from build123d import *

# Parameters (mm, degrees)
SKETCH1_W                                     = 40
SKETCH1_H                                     = 30
BOSS_EXTRUDE1_DEPTH                           = 10
SKETCH2_W                                     = 4.5
SKETCH2_H                                     = 8
CUT_EXTRUDE1_DEPTH                            = 1
CUT_EXTRUDE2_DEPTH                            = 11
SKETCH4_W                                     = 40
SKETCH4_H                                     = 15.897693
BOSS_EXTRUDE3_DEPTH                           = 15
FIX_DISTANCES_CONVEX_LENS_SEAT_DEPTH          = 3
CHOOSE_SCREW_SIZE_USE_TIGHT_TOLERANCE_C_DEPTH = 16.897693


with BuildPart() as part:
    # Sketch1 → Boss-Extrude1 (new body)
    with BuildSketch(Plane(origin=(0, 0, 0), x_dir=(0, 0, -1), z_dir=(1, 0, 0))):
        with Locations((3.569892473, -6.978494624)):
            Rectangle(SKETCH1_W, SKETCH1_H)
    extrude(amount=BOSS_EXTRUDE1_DEPTH)

    # Sketch2 → Cut-Extrude1 (cut)
    with BuildSketch(Plane.ZY):
        with BuildLine():
            Line((-5.319892473, 2.419198376), (-1.819892473, 2.419198376))
            ThreePointArc((-1.819892473, 2.419198376), (-1.466339083, 2.272751767), (-1.319892473, 1.919198376))
            Line((-1.319892473, 1.919198376), (-5.819892473, 1.919198376))
            ThreePointArc((-5.819892473, 1.919198376), (-5.673445864, 2.272751767), (-5.319892473, 2.419198376))
        make_face()
        with BuildLine():
            Line((-5.319892473, -6.580801624), (-1.819892473, -6.580801624))
            ThreePointArc((-1.819892473, -6.580801624), (-1.466339083, -6.434355014), (-1.319892473, -6.080801624))
            Line((-1.319892473, -6.080801624), (-5.819892473, -6.080801624))
            ThreePointArc((-5.819892473, -6.080801624), (-5.673445864, -6.434355014), (-5.319892473, -6.580801624))
        make_face()
        with Locations((-3.569892473, -2.080801624)):
            Rectangle(SKETCH2_W, SKETCH2_H)
        with BuildLine():
            ThreePointArc((-2.569892473, 2.419198376), (-3.569892473, 3.419198376), (-4.569892473, 2.419198376))
            Line((-4.569892473, 2.419198376), (-2.569892473, 2.419198376))
        make_face()
        with BuildLine():
            Line((-2.569892473, -6.580801624), (-4.569892473, -6.580801624))
            ThreePointArc((-4.569892473, -6.580801624), (-3.569892473, -7.580801624), (-2.569892473, -6.580801624))
        make_face()
    extrude(amount=-CUT_EXTRUDE1_DEPTH, mode=Mode.SUBTRACT)

    # Sketch3 → Cut-Extrude2 (cut, through all)
    with BuildSketch(Plane.ZY):
        with BuildLine():
            Line((-18.069892473, 1.919198376), (10.930107527, 1.919198376))
            ThreePointArc((10.930107527, 1.919198376), (12.69787448, 1.186965329), (13.430107527, -0.580801624))
            Line((13.430107527, -0.580801624), (13.430107527, -3.580801624))
            ThreePointArc((13.430107527, -3.580801624), (12.69787448, -5.348568577), (10.930107527, -6.080801624))
            Line((10.930107527, -6.080801624), (-18.069892473, -6.080801624))
            ThreePointArc((-18.069892473, -6.080801624), (-19.837659426, -5.348568577), (-20.569892473, -3.580801624))
            Line((-20.569892473, -3.580801624), (-20.569892473, -0.580801624))
            ThreePointArc((-20.569892473, -0.580801624), (-19.837659426, 1.186965329), (-18.069892473, 1.919198376))
        make_face()
    extrude(amount=-CUT_EXTRUDE2_DEPTH, mode=Mode.SUBTRACT)

    # Sketch4 → Boss-Extrude3 (add)
    with BuildSketch(Plane(origin=(10, 0, 0), x_dir=(0, 0, -1), z_dir=(1, 0, 0))):
        with Locations((3.569892473, -14.029648124)):
            Rectangle(SKETCH4_W, SKETCH4_H)
    extrude(amount=BOSS_EXTRUDE3_DEPTH)

    # Sketch6 → [fix distances] convex_lens_seat (cut)
    with BuildSketch(Plane(origin=(0, -6.080801624, 0), x_dir=(1, 0, 0), z_dir=(0, 1, 0))):
        Polygon((17, 2.569892473), (17, -1.680107527), (25, -1.680107527), (25, 8.819892473), (17, 8.819892473), (17, 4.569892473), align=None)
        with BuildLine():
            ThreePointArc((17, 4.569892473), (16, 3.569892473), (17, 2.569892473))
            Line((17, 2.569892473), (17, 4.569892473))
        make_face()
    extrude(amount=-FIX_DISTANCES_CONVEX_LENS_SEAT_DEPTH, mode=Mode.SUBTRACT)

    # Sketch7 → [choose screw size, use tight tolerance clearance diameter ] slots (cut, through all)
    with BuildSketch(Plane(origin=(0, -6.080801624, 0), x_dir=(1, 0, 0), z_dir=(0, 1, 0))):
        with BuildLine():
            Line((15.746714751, 12.781776292), (15.746714751, 19.608008654))
            ThreePointArc((15.746714751, 19.608008654), (17.5, 21.361293903), (19.253285249, 19.608008654))
            Line((19.253285249, 19.608008654), (19.253285249, 12.781776292))
            ThreePointArc((19.253285249, 12.781776292), (17.5, 11.028491043), (15.746714751, 12.781776292))
        make_face()
        with BuildLine():
            Line((15.746714751, -5.641991346), (15.746714751, -12.468223708))
            ThreePointArc((15.746714751, -12.468223708), (17.5, -14.221508957), (19.253285249, -12.468223708))
            Line((19.253285249, -12.468223708), (19.253285249, -5.641991346))
            ThreePointArc((19.253285249, -5.641991346), (17.5, -3.888706097), (15.746714751, -5.641991346))
        make_face()
    extrude(amount=-CHOOSE_SCREW_SIZE_USE_TIGHT_TOLERANCE_C_DEPTH, mode=Mode.SUBTRACT)


solid = part.part
Input: part model. Units: mm. Frame: model coordinates. A direction names the side the tool comes from. Give positions to 0.01 mm unless a question says otherwise; leave off trailing zeros. Write each loop counter-clockwise with the first axis right and the second up, starting at its lowest first coordinate (ties: lowest second). Pieces come first, ordered by that corner, then holes. Notation, with made-up numbers: (39, -13.5) -> (98, -13.5) arc R14 cw to (98, 3.5) -> close; hole circle Ø6 at (14, 4.25). An arc over 180 degrees is marked (long way). Use one line per item in the form item = value. Start each with the question number.
1) Section query D-D on z = -9.5. Return the cut outline in (x, y), then the cut area to 3 significant figures.
2) Section query C-C on y = -18.25. Return the cut outline in (x, z), then the cut area to 3 significant figures.
3) Set-up query: faces 1 (the flat face through (1, 3, -4)), 2 (the flat face through (17, -8, 0)), 3 (the cylindrical face through (4.93, -5.368, -19.818)), 4 (the cylindrical face through (17.54, -13.92, -11.03)). Return all of +Z, -Z, +X, -X, +Y, -Y with unobstructed straight access to the full face (end or side cutting, diameter ignored); none if empty.
4) Section query B-B on x = 17.5. Return the cut outline in (y, z).
5) Section query A-A on z = -16. Return the cut outline in (x, y).
6) Pin query (flat end, axial travel): pin 1 (1.5 mm diameter, centred on y = -7.5, z = -0.5, fed in from +X). Return the tip coordinate at first contact, or that it passes through.
7) Ray query, probe 1 along Y at (x, z) = (6, 3.5); probe 2 along X at (y, z) = (-18, -14); probe 3 along X at (y, z) = (4.25, -2). Return the intervals inside material, ascending. Write a range as from..to.
8) Draft query along Y for faces 5 (the flat face through (12, -21.978, -3)), 6 (the flat face through (5, -2, 13.43)), 7 (the cylindrical face through (4.93, 1.206, 12.678)), 8 (the flat face through (25, -14, -3)). Return one class per face: pulls with the +Y half, pulls with the -Y half, needs draft (parallel to the pull), parting line crosses it, or undercut.
Outcome:
q1.outline = (0, -21.98) -> (25, -21.98) -> (25, -6.08) -> (0, -6.08) -> close; (0, 1.92) -> (10, 1.92) -> (10, 8.02) -> (0, 8.02) -> close
q1.area = 458 mm^2
q2.outline = (0, -23.57) -> (25, -23.57) -> (25, 16.43) -> (0, 16.43) -> close; hole (15.75, -19.61) arc R1.75 ccw to (19.25, -19.61) -> (19.25, -12.78) arc R1.75 ccw to (15.75, -12.78) -> close; hole (15.75, 5.64) arc R1.75 ccw to (19.25, 5.64) -> (19.25, 12.47) arc R1.75 ccw to (15.75, 12.47) -> close
q2.area = 933 mm^2
q3.face_1 = -X
q3.face_2 = +X, +Y
q3.face_3 = +X, -X
q3.face_4 = +Y, -Y
q4.outline = (-21.98, -23.57) -> (-6.08, -23.57) -> (-6.08, -21.36) -> (-21.98, -21.36) -> close; (-21.98, -11.03) -> (-6.08, -11.03) -> (-6.08, -8.82) -> (-9.08, -8.82) -> (-9.08, 1.68) -> (-6.08, 1.68) -> (-6.08, 3.89) -> (-21.98, 3.89) -> close; (-21.98, 14.22) -> (-6.08, 14.22) -> (-6.08, 16.43) -> (-21.98, 16.43) -> close
q5.outline = (0, -21.98) -> (15.75, -21.98) -> (15.75, -6.08) -> (0, -6.08) -> close; (0, 1.92) -> (10, 1.92) -> (10, 8.02) -> (0, 8.02) -> close; (19.25, -21.98) -> (25, -21.98) -> (25, -6.08) -> (19.25, -6.08) -> close
q6.pin_1 = 17
q7.probe_1 = -21.98..-6.08, 1.92..8.02
q7.probe_2 = 0..15.75, 19.25..25
q7.probe_3 = 0..10
q8.face_5 = pulls with the -Y half
q8.face_6 = undercut
q8.face_7 = undercut
q8.face_8 = needs draft
